```python
from build123d import *

# Parameters (mm, degrees)
F0_W     = 59
F0_H     = 41.2
F1_DEPTH = 21.2
F2_R     = 11.5
F3_DEPTH = 8
F4_R     = 6.4
F5_DEPTH = 0.1
F6_W     = 13
F6_H     = 16
F7_DEPTH = 0.1
F8_R     = 6.15
F9_DEPTH = 0.2


with BuildPart() as f1:
    # F0 (on Top) → F1 (new body)
    with BuildSketch(Plane.XY):
        Rectangle(F0_W, F0_H)
    extrude(amount=F1_DEPTH)

    # F2 (on face) → F3 (join)
    with BuildSketch(Plane.XY.offset(21.2)):
        with Locations((16, 8.1)):
            Circle(F2_R)
    extrude(amount=F3_DEPTH)

    # F4 (on face) → F5 (join)
    with BuildSketch(Plane(origin=(0, 20.6, 0), x_dir=(-1, 0, 0), z_dir=(0, 1, 0))):
        with Locations((17.8, 11.7)):
            Circle(F4_R)
    extrude(amount=F5_DEPTH)

    # F6 (on face) → F7 (cut)
    with BuildSketch(Plane.XY.offset(21.2)):
        with Locations((-17.1, 6.7)):
            Rectangle(F6_W, F6_H)
    extrude(amount=-F7_DEPTH, mode=Mode.SUBTRACT)

    # F8 (on face) → F9 (join)
    with BuildSketch(Plane.XY.offset(21.2)):
        with Locations((-17.1, -10.45)):
            Circle(F8_R)
    extrude(amount=F9_DEPTH)


solid = f1.part
```
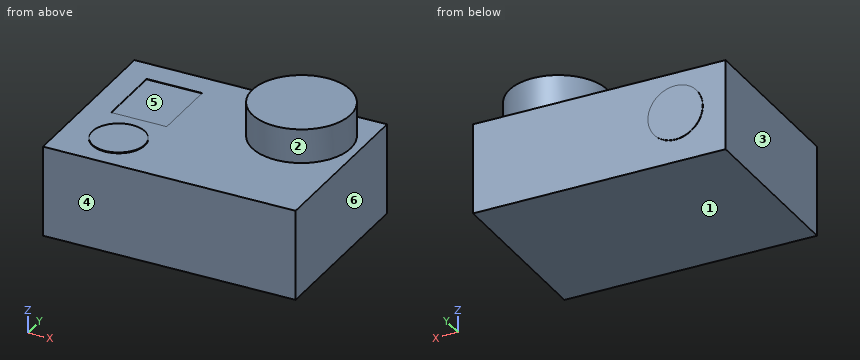
The model under review builds one solid part; all positions refer to its coordinate system, in mm. Face numbers are marked on the shaded views. A direction names the side the tool comes from. Give positions to 0.01 mm unless a question says otherwise; leave off trailing zeros. Write each loop counter-clockwise with the first axis right and the second up, starting at its lowest first coordinate (ties: lowest second). Pieces come first, ordered by that corner, then holes. Notation, with made-up numbers: M 32.5,12.5 L 72.5,12.5 A30 ccw 72.5,38.5 Z; hole C 6.25,61 d1. An arc over 180 degrees is marked long. Write item = value, one per line. Start each with the question number.
Q1. Machinability: for the marked faces 1 and 2, which of the approach directions +Z, -Z, +X, -X, +Y, -Y give a long, thin tool a straight path to every point of the face, cutting with its end or side? Answer none if there is none.
Q2. For line 1 (Z direction, x = -10, y = -6); line 2 (Y direction, x = -15.5, z = 1.5); line 3 (Z direction, x = -14.5, y = -1), list the stretches that pass through material, from the lowest coordinate up.
Q3. We need section C-C (z = 26.5). State the section outline as (x, y) points, plus the area to 3 significant figures.
Q4. We need section A-A (y = -10.45). State the section outline as (x, z) points, plus the area to 3 significant figures.
Q5. We need section B-B (x = 17.5). State the section outline as (y, z) points, plus the area to 3 significant figures.
Q6. We need section D-D (y = 8.1). State the section outline as (x, z) points, plus the area to 3 significant figures.
Q7. Clearance check with flat-ended pins moving along their axes: pin 1 (1.5 mm diameter, centred on x = 18, z = 15.5, fed in from +Y); pin 2 (14.5 mm diameter, centred on x = -19.5, y = 8.5, fed in from +Z); pin 3 (1 mm diameter, centred on x = -19.5, y = 6, fed in from +Z). State where each tip first meets the part, or that it passes through.
Q8. Mouldability with a two-part tool opening along X and no side actions: class the marked faces 3, 4, 5 and 6 as released by +X, released by -X, zero draft, split by the parting line, or undercut.
Result set:
q1.face_1 = -Z, +X, -X, +Y, -Y
q1.face_2 = +Z
q2.line_1 = 0 to 21.2
q2.line_2 = -20.6 to 20.6
q2.line_3 = 0 to 21.1
q3.outline = C 16,8.1 d23
q3.area = 415 mm2
q4.outline = M -29.5,0 L 29.5,0 L 29.5,21.2 L -10.95,21.2 L -10.95,21.4 L -23.25,21.4 L -23.25,21.2 L -29.5,21.2 Z
q4.area = 1,250 mm2
q5.outline = M -20.6,0 L 20.6,0 L 20.6,21.2 L 19.5,21.2 L 19.5,29.2 L -3.3,29.2 L -3.3,21.2 L -20.6,21.2 Z
q5.area = 1,060 mm2
q6.outline = M -29.5,0 L 29.5,0 L 29.5,21.2 L 27.5,21.2 L 27.5,29.2 L 4.5,29.2 L 4.5,21.2 L -10.6,21.2 L -10.6,21.1 L -23.6,21.1 L -23.6,21.2 L -29.5,21.2 Z
q6.area = 1,430 mm2
q7.pin_1 = 20.6
q7.pin_2 = 21.2
q7.pin_3 = 21.1
q8.face_3 = released by -X
q8.face_4 = zero draft
q8.face_5 = undercut
q8.face_6 = released by +X
